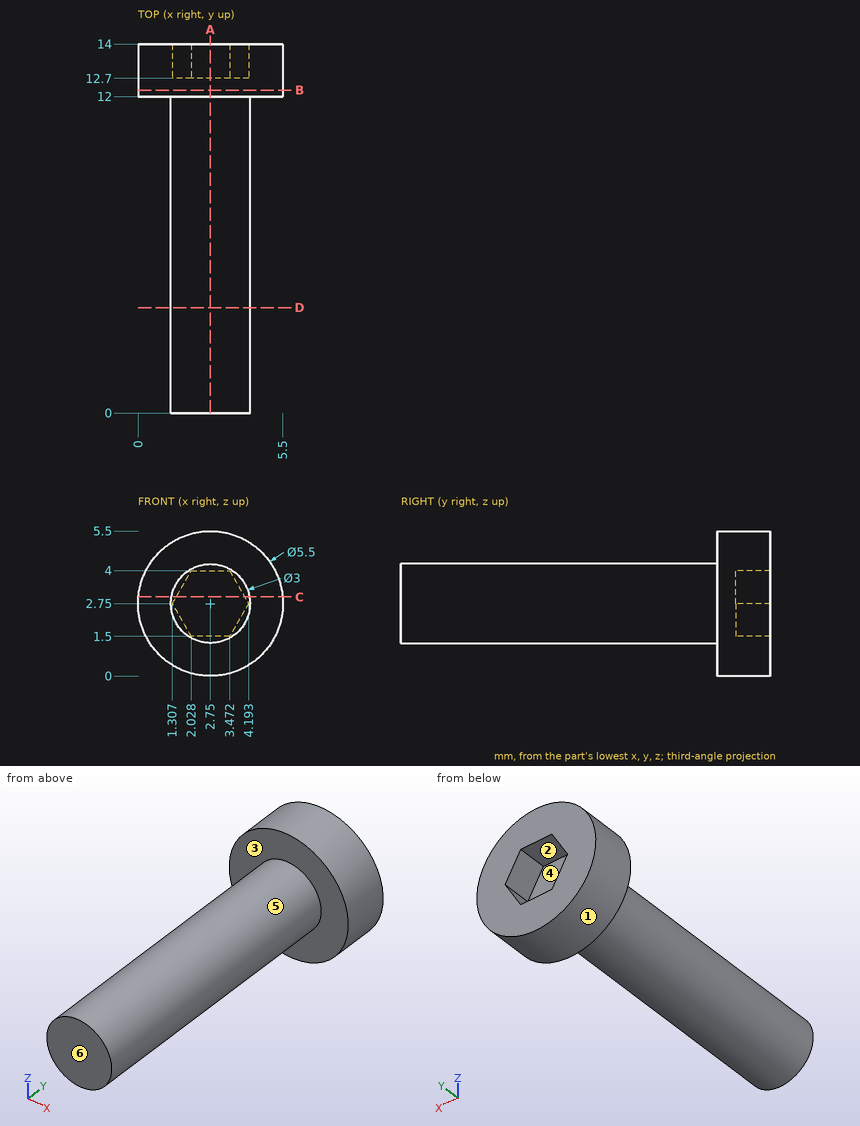
Could you check a few things on this drawing? It's one solid part, dimensions in mm from its lowest x, y, z. A direction names the side the tool comes from. Give positions to 0.01 mm unless a question says otherwise; leave off trailing zeros. Order: outer loops, then holes, each group sorted by start corner. A loop starts at its lowest first (then second) coordinate and runs counter-clockwise, first axis right, second up. Notation, with made-up numbers: (11, -24) -> (19, -24) arc R29 cw to (19, 15) -> close; hole circle Ø7 at (48.5, 59). An arc over 180 degrees is marked (long way). Use CSV: the item, a comma, the result in double quotes. Start each with the question number.
Item 1: I'm going to push flat-ended pins straight in: P1, Ø1.5, axis at y = 5.5, z = 1, coming from the +X side; P2, Ø1.5, axis at y = 9, z = 2.5, coming from the +X side. Where does each tip first touch, or does it pass through?
Item 2: Thinking about a two-plate mould opening in Z: for the marked faces 4, 5 and 6, which applies, pulls with the +Z half, pulls with the -Z half, needs draft (parallel to the pull), parting line crosses it, or undercut?
Item 3: If I drill on probe 1 along Y at (x, z) = (2.65, 2.6); probe 2 along Y at (x, z) = (4.5, 3.6); probe 3 along Z at (x, y) = (2.35, 0.5) (1 decimal), over which ranges is the centre line in solid material (lowest first)? Write a range as [from, to].
Item 4: Suppose I cut it at A-A (x = 2.75). List the corners of the cut face in (y, z) for me.
Item 5: Suppose I cut it at B-B (y = 12.25). List the corners of the cut face in (x, z) for me.
Item 6: Suppose I cut it at C-C (z = 3). List the corners of the cut face in (x, y) for me.
Item 7: Suppose I cut it at D-D (y = 4). List the corners of the cut face in (x, z) for me.
Item 8: On a 3-axis mill with a long thin cutter (end or side, diameter ignored), from which of +Z, -Z, +X, -X, +Y, -Y can I reach the whole of each face in a straight line? I mean the marked faces 1, 2 and 3. Say none if no direction works.
Answer block:
1,P1,"stops at x = 3.87"
1,P2,"stops at x = 4.25"
2,face 4,"undercut"
2,face 5,"parting line crosses it"
2,face 6,"needs draft"
3,probe 1,"y = [0, 12.7]"
3,probe 2,"y = [12, 14]"
3,probe 3,"z = [1.3, 4.2]"
4,outline,"(0, 1.25) -> (12, 1.25) -> (12, 0) -> (14, 0) -> (14, 1.5) -> (12.7, 1.5) -> (12.7, 4) -> (14, 4) -> (14, 5.5) -> (12, 5.5) -> (12, 4.25) -> (0, 4.25) -> close"
5,outline,"circle Ø5.5 at (2.75, 2.75)"
6,outline,"(0.01, 12) -> (1.27, 12) -> (1.27, 0) -> (4.23, 0) -> (4.23, 12) -> (5.49, 12) -> (5.49, 14) -> (4.05, 14) -> (4.05, 12.7) -> (1.45, 12.7) -> (1.45, 14) -> (0.01, 14) -> close"
7,outline,"circle Ø3 at (2.75, 2.75)"
8,face 1,"+Y, -Y"
8,face 2,"+Y"
8,face 3,"-Y"
